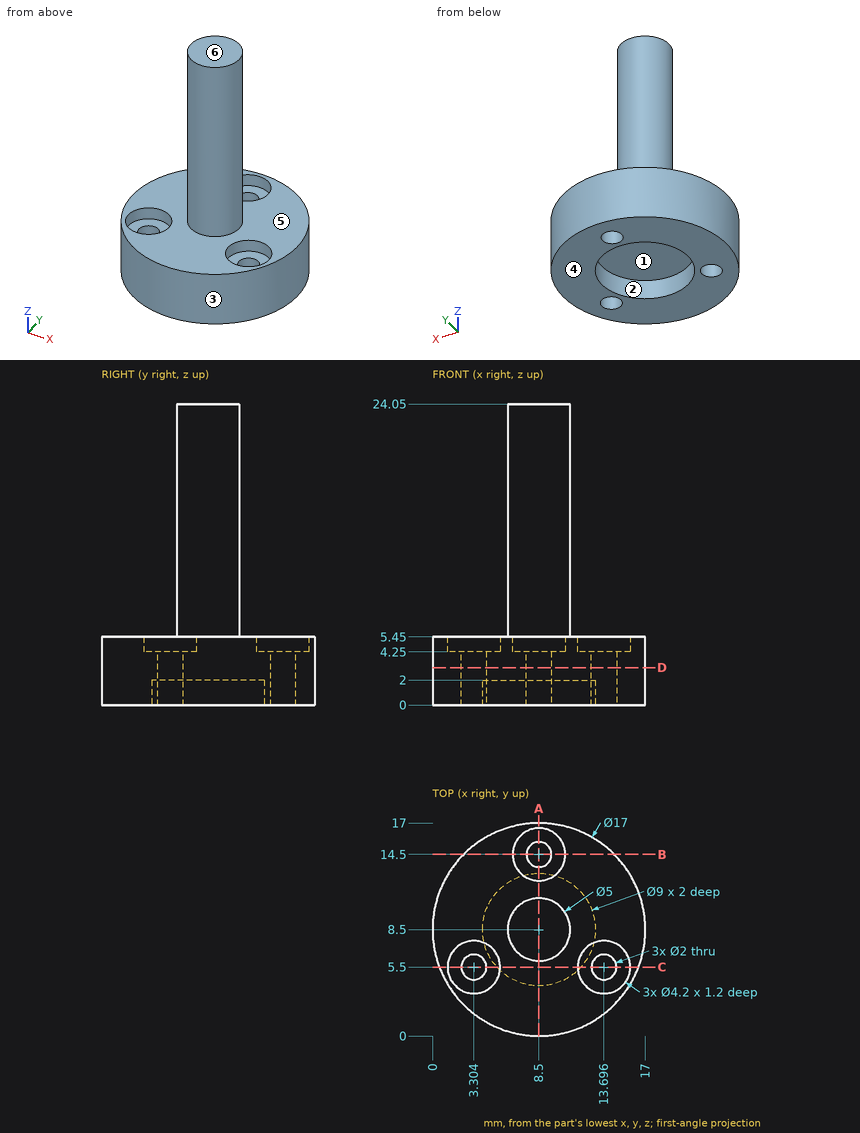
The drawing under review shows one solid part. Ordinate dimensions are in mm from its lowest x, y, z. A direction names the side the tool comes from. Coordinates: 2 decimals unless noted, no trailing zeros. Write each loop counter-clockwise with the first axis right and the second up, starting at its lowest first coordinate (ties: lowest second). Pieces come first, ordered by that corner, then holes. Notation, with made-up numbers: (55, -11) - (97, -11) arc R23 cw to (97, 2) - close; hole circle Ø1 at (20, 14). An arc over 180 degrees is marked (long way). Put each result on its own line as item: value.
1. For pin 1 (3.5 mm diameter, centred on x = 3, y = 5, fed in from +Z); pin 2 (6 mm diameter, centred on x = 4.5, z = 3.5, fed in from +Y); pin 3 (10 mm diameter, centred on y = 12.5, z = 21, fed in from +X); pin 4 (6 mm diameter, centred on y = 2.5, z = 10.5, fed in from +X), all flat-tipped, find the tip position at first contact; note any pin that passes through.
Values found:
pin 1: z = 5.45
pin 2: y = 16.94
pin 3: x = 11
pin 4: through
2. Mouldability with a two-part tool opening along X and no side actions: class the marked faces 1, 2, 3 and 4 as released by +X, released by -X, zero draft, split by the parting line, or undercut.
Values found:
face 1: undercut
face 2: undercut
face 3: split by the parting line
face 4: zero draft
3. Add section A-A, the plane x = 8.5. Give the boundary of the cut face in (y, z).
Values found:
outline: (0, 0) - (4, 0) - (4, 2) - (13, 2) - (13, 0) - (13.5, 0) - (13.5, 4.25) - (12.4, 4.25) - (12.4, 5.45) - (11, 5.45) - (11, 24.05) - (6, 24.05) - (6, 5.45) - (0, 5.45) - close; (15.5, 0) - (17, 0) - (17, 5.45) - (16.6, 5.45) - (16.6, 4.25) - (15.5, 4.25) - close
4. Add section D-D, the plane z = 3. Give the boundary of the cut face in (x, y).
Values found:
outline: circle Ø17 at (8.5, 8.5); hole circle Ø2 at (3.3, 5.5); hole circle Ø2 at (8.5, 14.5); hole circle Ø2 at (13.7, 5.5)
5. Add section B-B, the plane y = 14.5. Give the boundary of the cut face in (x, z).
Values found:
outline: (2.48, 0) - (7.5, 0) - (7.5, 4.25) - (6.4, 4.25) - (6.4, 5.45) - (2.48, 5.45) - close; (9.5, 0) - (14.52, 0) - (14.52, 5.45) - (10.6, 5.45) - (10.6, 4.25) - (9.5, 4.25) - close
6. Wall thickness on probe 1 along Y at (x, z) = (8.5, 0.9); probe 2 along Y at (x, z) = (8.5, 3); probe 3 along Y at (x, z) = (1.5, 5.25) (1 decimal): over which ranges is each line inside the solid? List them lowest first.
Values found:
probe 1: 0 to 4, 13 to 13.5, 15.5 to 17
probe 2: 0 to 13.5, 15.5 to 17
probe 3: 3.7 to 4.4, 6.6 to 13.3
7. Machinability: for the marked faces 5 and 6, which of the approach directions +Z, -Z, +X, -X, +Y, -Y give a long, thin tool a straight path to every point of the face, cutting with its end or side? Answer none if there is none.
Values found:
face 5: +Z
face 6: +Z, +X, -X, +Y, -Y
8. Add section C-C, the plane y = 5.5. Give the boundary of the cut face in (x, z), then the cut area to 3 significant figures.
Values found:
outline: (0.55, 0) - (2.3, 0) - (2.3, 4.25) - (1.2, 4.25) - (1.2, 5.45) - (0.55, 5.45) - close; (4.3, 0) - (5.15, 0) - (5.15, 2) - (11.85, 2) - (11.85, 0) - (12.7, 0) - (12.7, 4.25) - (11.6, 4.25) - (11.6, 5.45) - (5.4, 5.45) - (5.4, 4.25) - (4.3, 4.25) - close; (14.7, 0) - (16.45, 0) - (16.45, 5.45) - (15.8, 5.45) - (15.8, 4.25) - (14.7, 4.25) - close
area: 46.2 mm²
